Autodesk Inventor part; units mm, degrees
ref_plane "YZ Plane" through (0, 0, 0) normal (1, 0, 0) x (0, 1, 0)
ref_plane "XZ Plane" through (0, 0, 0) normal (0, 1, 0) x (-1, 0, 0)
ref_plane "XY Plane" through (0, 0, 0) normal (0, 0, 1) x (1, 0, 0)
sketch "Sketch1" plane through (0, 0, 0) normal (0, 1, 0) x (-1, 0, 0)
  line L0 (0, 0) -> (69, 0)
  line L1 (69, 0) -> (69, -65)
  line L2 (69, -65) -> (0, -65)
  line L3 (0, -65) -> (0, 0)
  dimension "d0" = 69
  dimension "d1" = 65
extrude "Extrusion1" add sketch "Sketch1" along normal blind 3
sketch "Sketch2" plane through (0, 3, 0) normal (0, 1, 0) x (1, 0, 0)
  line L0 (0, 65) -> (-69, 65)
  line L1 (-69, 65) -> (-66, 65)
  line L2 (-66, 65) -> (-66, 0)
  line L3 (-66, 0) -> (-69, 0)
  line L4 (-69, 0) -> (-69, 65)
  point P0 (0, 0)
  dimension "d4" = 3
  dimension "d5" = 65
extrude "Extrusion2" add sketch "Sketch2" along normal blind 66
fillet "Fillet1" radius 2 2 edges at (-66, 3, -32.5) (-69, 0, -32.5)
sketch "Sketch3" plane through (0, 0, 0) normal (0, 0, 1) x (1, 0, 0)
  line L0 (-67, 0) -> (0, 0)
  line L1 (-66, 0) -> (-51, 0) construction
  line L2 (-66, 5) -> (-66, 69)
  line L3 (-66, 5) -> (-66, 0)
  line L4 (-66, 5) -> (-61, 5) construction
  line L5 (-66, 0) -> (-51, 0)
  line L6 (-66, 0) -> (-66, 25)
  line L7 (-66, 25) -> (-51, 0)
  dimension "d12" = 5
  dimension "d13" = 90
  dimension "d14" = 15
  dimension "d15" = 90
  dimension "d16" = 25
extrude "Extrusion3" add sketch "Sketch3" against normal blind 3
pattern_linear "Rectangular Pattern1" count 2 spacing 62 along (0, 0, -1) of "Extrusion3"
sketch "Sketch4" plane through (-66, 69, 0) normal (1, 0, 0) x (0, 0, -1)
  circle A0 centre (32.5, -29) radius 22.5
  line L0 (0, 0) -> (65, 0)
  line L1 (0, -44) -> (0, 0)
  point P0 (0, -69)
  dimension "d22" = 45
  dimension "d23" = 29
  dimension "d24" = 32.5
extrude "Extrusion4" cut sketch "Sketch4" against normal blind 3
sketch "Sketch5" plane through (-66, 69, 0) normal (1, 0, 0) x (0, 0, -1)
  circle A0 centre (9, -5.501) radius 2.6
  line L0 (0, 0) -> (65, 0)
  line L1 (0, -44) -> (0, 0)
  circle A1 centre (56, -5.501) radius 2.6
  circle A2 centre (9, -52.501) radius 2.6
  circle A3 centre (56, -52.501) radius 2.6
  point P0 (0, -69)
  dimension "d27" = 5.2
  dimension "d28" = 5.501
  dimension "d29" = 9
  dimension "d32" = 47
  dimension "d35" = 47
extrude "Extrusion5" cut sketch "Sketch5" against normal blind 3
sketch "Sketch6" plane through (0, 3, 0) normal (0, 1, 0) x (1, 0, 0)
  line L0 (-52.8, 0) -> (0, 0)
  line L1 (0, 0) -> (0, 65)
  arc A0 (-10, 10.4) -> (-10, 14.6) centre (-10, 12.5) ccw
  arc A1 (-52, 14.6) -> (-52, 10.4) centre (-52, 12.5) ccw
  line L2 (-10, 14.6) -> (-52, 14.6)
  line L3 (-69, 65) -> (-69, 0)
  line L4 (-10, 12.5) -> (-7.9, 12.5) construction
  line L5 (-10, 10.4) -> (-52, 10.4)
  dimension "d47" = 4.2
  dimension "d48" = 4.2
  dimension "d49" = 12.5
  dimension "d50" = 12.5
  dimension "d52" = 42
  dimension "d54" = 17
extrude "Extrusion6" cut sketch "Sketch6" against normal blind 3
pattern_linear "Rectangular Pattern2" count 2 spacing 40 along (0, 0, -1) of "Extrusion6"
properties part number "NEMA23_StepperonlineMount"
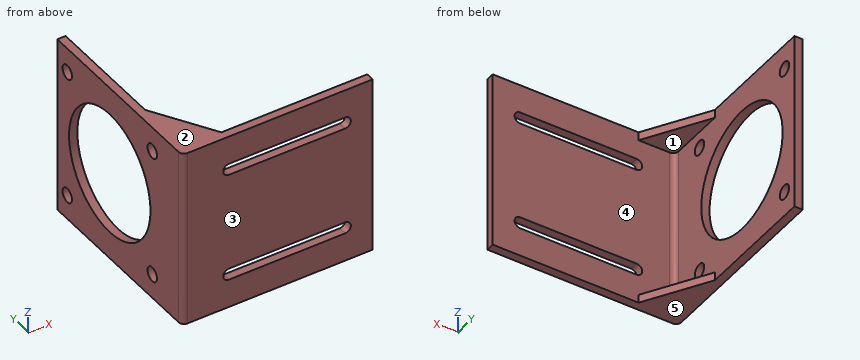
Design review of the part built by this model. Coordinates are the model's own, in mm. Face numbers are marked on the shaded views. A direction names the side the tool comes from. Round coordinates to 2 decimals unless told otherwise and drop trailing zeros. Order: outer loops, then holes, each group sorted by start corner. A loop starts at its lowest first (then second) coordinate and runs counter-clockwise, first axis right, second up. Notation, with made-up numbers: (58, 83.5) - (82, 83.5) arc R22 ccw to (82, 101.5) - close; hole circle Ø5 at (1.25, 9.25). An arc over 180 degrees is marked (long way). Return JSON: item names as keys, results as strings.
Q1. Machinability: for the marked faces 4 and 5, which of the approach directions +Z, -Z, +X, -X, +Y, -Y give a long, thin tool a straight path to every point of the face, cutting with its end or side? Answer none if there is none.
Computed values:
{"face 4": "+X, +Y", "face 5": "-Z, +X, -X, +Y, -Y"}
Q2. Consider section B-B on y = 40. Write out the cut boundary in (x, z), plus the area to 3 significant figures.
Computed values:
{"outline": "(-69, -65) - (-66, -65) - (-66, -55) - (-69, -55) - close; (-69, -10) - (-66, -10) - (-66, 0) - (-69, 0) - close", "area": "60.0 mm2"}
Q3. Consider section D-D on z = -24. Write out the cut boundary in (x, y).
Computed values:
{"outline": "(-69, 2) arc R2 ccw to (-67, 0) - (0, 0) - (0, 3) - (-64, 3) arc R2 cw to (-66, 5) - (-66, 19.17) - (-69, 19.17) - close; (-69, 60.83) - (-66, 60.83) - (-66, 69) - (-69, 69) - close"}
Q4. Wall thickness on L1, parallel to Y at x = -67, z = -56; L2, parallel to X at y = 66.5, z = -59; L3, parallel to Y at x = -60, z = -56: over which ranges is each line inside the solid? List them lowest first. Write a range as [from, to].
Computed values:
{"L1": "y = [0, 13.9], [19.1, 60.9], [66.1, 69]", "L2": "x = [-69, -66]", "L3": "y = [0, 3]"}
Q5. For pin 1 Ø1 at (x, z) = (-44.5, -20.5) entering from -Y; pin 2 Ø3 at (x, z) = (-23.5, -41) entering from +Y; pin 3 Ø8.5 at (y, z) = (63.499, -9) entering from +X; pin 4 Ø3 at (y, z) = (16.499, -56) entering from +X, all flat-tipped, find the tip position at first contact; note any pin that passes through.
Computed values:
{"pin 1": "stops at y = 0", "pin 2": "stops at y = 3", "pin 3": "stops at x = -66", "pin 4": "passes through"}
Q6. Consider section C-C on x = -49.5. Write out the cut boundary in (y, z), plus the area to 3 significant figures.
Computed values:
{"outline": "(0, -65) - (3, -65) - (3, -54.6) - (0, -54.6) - close; (0, -50.4) - (3, -50.4) - (3, -14.6) - (0, -14.6) - close; (0, -10.4) - (3, -10.4) - (3, 0) - (0, 0) - close", "area": "170 mm2"}
Q7. Consider section A-A on z = -9. Write out the cut boundary in (x, y), plus the area to 3 significant figures.
Computed values:
{"outline": "(-69, 2) arc R2 ccw to (-67, 0) - (0, 0) - (0, 3) - (-64, 3) arc R2 cw to (-66, 5) - (-66, 13.9) - (-69, 13.9) - close; (-69, 19.1) - (-66, 19.1) - (-66, 60.9) - (-69, 60.9) - close; (-69, 66.1) - (-66, 66.1) - (-66, 69) - (-69, 69) - close", "area": "374 mm2"}
Q8. The part is to be moulded in two halves that separate along Z. For the marked faces 1, 2 and 3, say which applies: pulls with the +Z half, pulls with the -Z half, needs draft (parallel to the pull), parting line crosses it, or undercut.
Computed values:
{"face 1": "undercut", "face 2": "pulls with the +Z half", "face 3": "needs draft"}
